Here's the drawing with two shaded views (mm, measured from the low corner). I have some questions. A direction names the side the tool comes from. Give positions to 0.01 mm unless a question says otherwise; leave off trailing zeros. Loops run counter-clockwise (first coordinate to the right, second up) from the corner with the lowest first, then second, coordinate; pieces in that order, holes last.
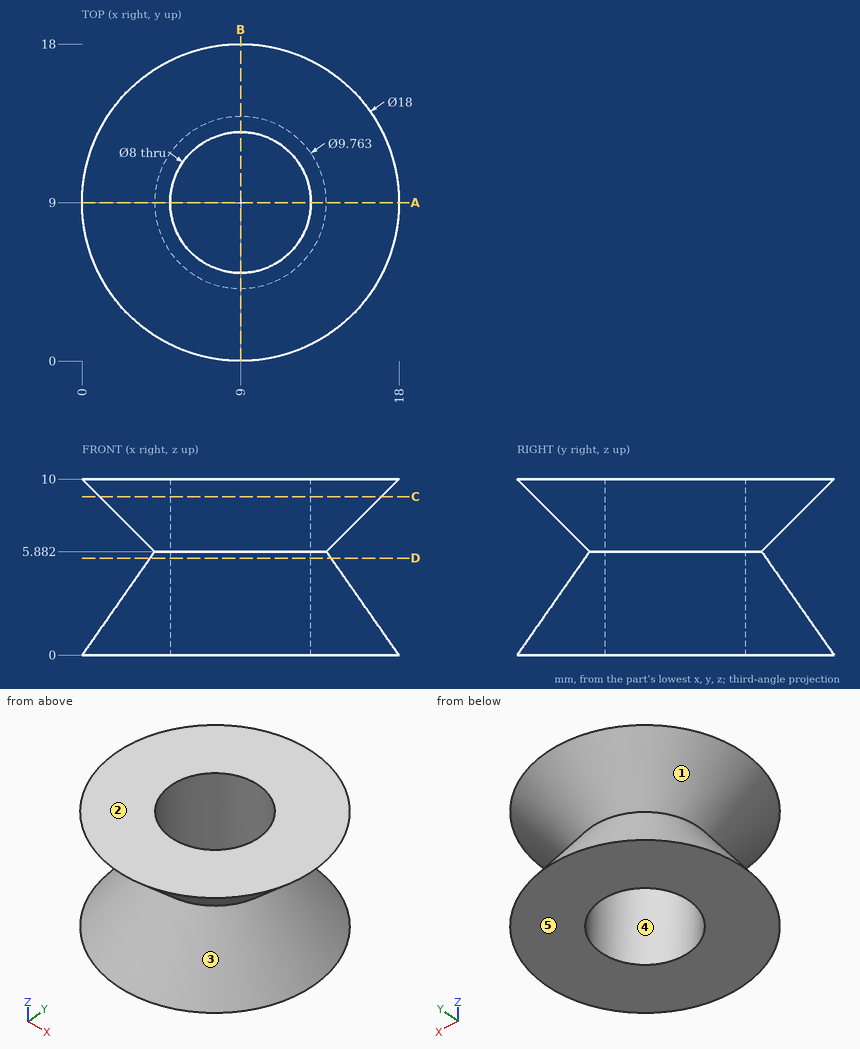
(1) Suppose I cut it at D-D on z = 5.5. List the corners of the cut face in (x, y) for me.
Returned:
outline: circle Ø10.3 at (9, 9); hole circle Ø8 at (9, 9)
(2) Thinking about a two-plate mould opening in Z: for the marked faces 3, 4 and 5, which applies, pulls with the +Z half, pulls with the -Z half, needs draft (parallel to the pull), parting line crosses it, or undercut?
Returned:
face 3: undercut
face 4: needs draft
face 5: pulls with the -Z half
(3) Will these pins go through, and if not, where does the flat tip stop? P1, Ø1.5, axis at y = 7.5, z = 8.5, coming from the +X side (1 decimal); P2, Ø3, axis at y = 4, z = 7.5, coming from the +X side; P3, Ø4, axis at y = 5, z = 1.5, coming from the +X side.
Returned:
P1: stops at x = 17.1
P2: stops at x = 15.54
P3: stops at x = 17.59
(4) Please list where these lines run through material, in increasing order: probe 1 along Z at (x, y) = (15.5, 6.5) (1 decimal); probe 2 along X at (y, z) = (6.25, 1.5) (1 decimal); probe 3 along X at (y, z) = (7.5, 6.25).
Returned:
probe 1: z = 0 to 2.9, 8 to 10
probe 2: x = 1.5 to 6.1, 11.9 to 16.5
probe 3: x = 3.97 to 5.29, 12.71 to 14.03
(5) Suppose I cut it at C-C on z = 9. List the corners of the cut face in (x, y) for me, plus the area to 3 significant figures.
Returned:
outline: circle Ø16 at (9, 9); hole circle Ø8 at (9, 9)
area: 151 mm2
(6) Which directions (+Z, -Z, +X, -X, +Y, -Y) give clear straight access to the entire face, cutting with the end or side of a thin tool? Please do the marked faces 1 and 2.
Returned:
face 1: none
face 2: +Z, +X, -X, +Y, -Y
(7) Suppose I cut it at A-A on y = 9. List the corners of the cut face in (x, z) for me.
Returned:
outline: (0, 0) - (5, 0) - (5, 10) - (0, 10) - (4.12, 5.88) - close; (13, 0) - (18, 0) - (13.88, 5.88) - (18, 10) - (13, 10) - close
